from build123d import *

# Parameters (mm, degrees)
SKETCH_1_W          = 30
SKETCH_1_H          = 28
EXTRUDE_1_DEPTH     = 5
CUT_EXTRUDE_1_DEPTH = 22.118712082
SKETCH_3_W          = 30
SKETCH_3_H          = 5
EXTRUDE_2_DEPTH     = 35
FILLET_1_R          = 5
FILLET_2_R          = 15
FILLET_3_R          = 15
SKETCH_4_R          = 10
CUT_EXTRUDE_2_DEPTH = 49.518037883
FILLET_5_R          = 5


with BuildPart() as part:
    # Эскиз1 → Бобышка-Вытянуть1 (new body)
    with BuildSketch(Plane.XY):
        Rectangle(SKETCH_1_W, SKETCH_1_H)
    extrude(amount=EXTRUDE_1_DEPTH)

    # Эскиз2 → Вырез-Вытянуть1 (cut, through all)
    with BuildSketch(Plane.XY.offset(5)):
        with BuildLine():
            Line((-6, 14), (6, 14))
            Line((6, 14), (6, 4))
            ThreePointArc((6, 4), (0, -2), (-6, 4))
            Line((-6, 4), (-6, 14))
        make_face()
    extrude(amount=-CUT_EXTRUDE_1_DEPTH, mode=Mode.SUBTRACT)

    # Эскиз3 → Бобышка-Вытянуть2 (add)
    with BuildSketch(Plane.XY.offset(5)):
        with Locations((0, -11.5)):
            Rectangle(SKETCH_3_W, SKETCH_3_H)
    extrude(amount=EXTRUDE_2_DEPTH)

    # Скругление1
    fillet_1_edges = [part.edges().sort_by_distance(p)[0] for p in [
        (0, -14, 0),
    ]]
    fillet(fillet_1_edges, radius=FILLET_1_R)

    # Скругление2
    fillet_2_edges = [part.edges().sort_by_distance(p)[0] for p in [
        (15, -11.5, 40),
    ]]
    fillet(fillet_2_edges, radius=FILLET_2_R)

    # Скругление3
    fillet_3_edges = [part.edges().sort_by_distance(p)[0] for p in [
        (-15, -11.5, 40),
    ]]
    fillet(fillet_3_edges, radius=FILLET_3_R - 0.0001)  # a hair under: the kernel refuses the full size

    # Эскиз4 → Вырез-Вытянуть2 (cut, through all)
    with BuildSketch(Plane(origin=(0, -9, 0), x_dir=(1, 0, 0), z_dir=(0, 1, 0))):
        with Locations(Location((0, -25, 0), (0, 0, 270))):
            Circle(SKETCH_4_R)
    extrude(amount=-CUT_EXTRUDE_2_DEPTH, mode=Mode.SUBTRACT)

    # Скругление5
    fillet_5_edges = [part.edges().sort_by_distance(p)[0] for p in [
        (0, -9, 5),
    ]]
    fillet(fillet_5_edges, radius=FILLET_5_R)


solid = part.part
Verification items for the finished model (mm, model axes). A direction names the side the tool comes from. Coordinates: 2 decimals unless noted, no trailing zeros. Loops run counter-clockwise (first coordinate to the right, second up) from the corner with the lowest first, then second, coordinate; pieces in that order, holes last. Notation, with made-up numbers: M 22.5,-22.5 L 47.5,-22.5 A21 cw 47.5,-14.5 Z; hole C 68.25,87 d9. An arc over 180 degrees is marked long. One line per item, written item: value.
1. Section check A-A on y = 7.5. Record the cut outline in (x, z), plus the area to 3 significant figures.
Answers follow:
outline: M -15,0 L -6,0 L -6,5 L -15,5 Z; M 6,0 L 15,0 L 15,5 L 6,5 Z
area: 90.0 mm^2
2. Section check C-C on z = 23. Record the cut outline in (x, y), plus the area to 3 significant figures.
Answers follow:
outline: M -15,-14 L -9.8,-14 L -9.8,-9 L -15,-9 Z; M 9.8,-14 L 15,-14 L 15,-9 L 9.8,-9 Z
area: 52.0 mm^2
3. Section check D-D on x = -9. Record the cut outline in (y, z).
Answers follow:
outline: M -14,5 A5 ccw -9,0 L 14,0 L 14,5 L -4,5 A5 cw -9,10 L -9,20.64 L -14,20.64 Z; M -14,29.36 L -9,29.36 L -9,37 L -14,37 Z
4. Gauge pin test, flat ends, axial feed: P1, Ø6, axis at x = 7, y = -9.5, coming from the +Z side; P2, Ø4, axis at x = -6.5, y = 2.5, coming from the +Z side; P3, Ø16, axis at x = 0, z = 25, coming from the +Y side. Record the tip position at first contact, or that the pin passes through.
Answers follow:
P1: z = 39.46
P2: z = 5
P3: through
5. Mould release check, pull along X, two halves, no side actions. Record for faces 3 (the cylindrical face through (0, -13, 2)), 4 (the cylindrical face through (-10.49, -11.46, 35.72)), 5 (the flat face through (-6, 9, 3)), 6 (the flat face through (6, 9, 3)): pulls with the +X half, pulls with the -X half, needs draft (parallel to the pull), parting line crosses it, or undercut.
Answers follow:
face 3: needs draft
face 4: pulls with the -X half
face 5: undercut
face 6: undercut
6. Section check B-B on x = -3.5. Record the cut outline in (y, z), plus the area to 3 significant figures.
Answers follow:
outline: M -14,5 A5 ccw -9,0 L -0.87,0 L -0.87,5 L -4,5 A5 cw -9,10 L -9,15.63 L -14,15.63 Z; M -14,34.37 L -9,34.37 L -9,39.59 L -14,39.59 Z
area: 145 mm^2
7. Set-up check for faces 1 (the flat face through (-0.2, -9, 14.8)), 2 (the cylindrical face through (3, -11.46, 34.54)): record each of +Z, -Z, +X, -X, +Y, -Y from which the full face is reachable in a straight line by a thin tool's end or side.
Answers follow:
face 1: +Z, +X, -X, +Y
face 2: +Y, -Y
8. Material ranges on line 1 along Z through (x, y) = (-2.5, -2.75); line 2 along Y through (x, z) = (-5.5, 10); line 3 along Z through (x, y) = (-8, -10), recorded low to high. Write a range as from..to.
Answers follow:
line 1: 0..5
line 2: -14..-9
line 3: 0.1..19, 31..37.69
